Build history of the part. All positions in model axes, mm. Coordinates: 2 decimals unless noted, no trailing zeros. Order: outer loops, then holes, each group sorted by start corner. A loop starts at its lowest first (then second) coordinate and runs counter-clockwise, first axis right, second up. Notation, with made-up numbers: (82.5, 32) - (108.5, 32) arc R8 cw to (108.5, 44) - close; hole circle Ø7 at (59.5, 36). An arc over 180 degrees is marked (long way). Return JSON: item names as keys, results as strings.
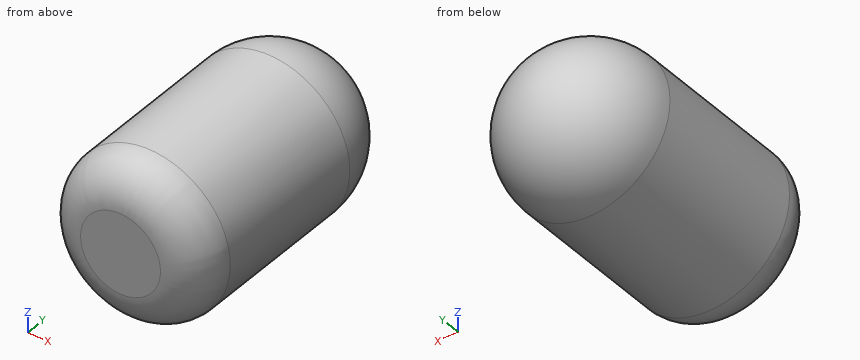
Autodesk Inventor part; units mm, degrees
ref_plane "YZ Plane" through (0, 0, 0) normal (1, 0, 0) x (0, 1, 0)
ref_plane "XZ Plane" through (0, 0, 0) normal (0, 1, 0) x (-1, 0, 0)
ref_plane "XY Plane" through (0, 0, 0) normal (0, 0, 1) x (1, 0, 0)
sketch "Sketch1" plane through (0, 0, 0) normal (0, 1, 0) x (-1, 0, 0)
  circle A0 centre (0, 0) radius 12.7
  point P0 (0, -12.7)
  dimension "d0" = 25.4
extrude "Extrusion1" add sketch "Sketch1" along normal blind 44.45
fillet "Fillet1" radius 12.7 1 edges at (12.7, 44.45, 0)
fillet "Fillet2" radius 6.35 1 edges at (12.7, 0, 0)
properties part number "minion-body" material "PAEK Plastic"
1. Drop flat-ended pins along their axis: pin 1 (2 mm diameter, centred on x = -2, y = 31.5, fed in from -Z); pin 2 (10 mm diameter, centred on x = 8, y = 35.5, fed in from +Z); pin 3 (1 mm diameter, centred on x = 8.5, z = -3, fed in from +Y). Give the stop position or say it passes through.
Check values:
{"pin 1": "z = -12.66", "pin 2": "z = 12.11", "pin 3": "y = 41.17"}
2. Cut at A-A on y = 27. Give the cut face in (x, z), plus the area to 3 significant figures.
Check values:
{"outline": "circle Ø25.4 at (0, 0)", "area": "507 mm²"}
3. Cut at B-B on y = 37. Give the cut face in (x, z), plus the area to 3 significant figures.
Check values:
{"outline": "circle Ø23.13 at (0, 0)", "area": "420 mm²"}
4. Probe L1, parallel to X at y = 24.5, z = 0.5; L2, parallel to X at y = 10.5, z = 2.5; L3, parallel to Z at x = 11, y = 27.5. List the from-to ranges inside material, lowest first.
Check values:
{"L1": "-12.69 to 12.69", "L2": "-12.45 to 12.45", "L3": "-6.35 to 6.35"}
